Can you work these out from the model? Positions are in its coordinate system, mm. Coordinates: 2 decimals unless noted, no trailing zeros. Order: outer loops, then holes, each group sorted by start corner. A loop starts at its lowest first (then second) coordinate and runs counter-clockwise, first axis right, second up. Notation, with made-up numbers: M 1,-14.75 L 57,-14.75 A31 ccw 57,23.25 Z; hole C 82.5,68.5 d1. An arc over 180 degrees is marked long. Answer as CSV lines item,"result". Start each with the question number.
1. Will this pin go through, and if not, where does the flat tip stop? pin 1 (8 mm diameter, centred on x = -0.5, y = 7.5, fed in from -Z).
2. If we section it at A-A (x = 0): List the corners of the cut face in (y, z) for me, plus the area to 3 significant figures.
3. If we mould it in two halves opening along Y, with no side actions, what happens to faces 1 (the face through (0, -20.5, 3)), 2 (the face through (-10.316, 7.91, 3.328)), 3 (the face through (-14.753, 20.383, 3.328))? For each: released by +Y, released by -Y, zero draft, split by the parting line, or undercut.
4. I need wall thicknesses on line 1 along Y through (x, z) = (0.5, 0.5); line 2 along Y through (x, z) = (16.5, 3); line 3 along Y through (x, z) = (-15.5, 5). Which ranges of each line are inside material? Lowest first, please. Write a range as from..to.
5. If we section it at C-C (z = 5.75): List the corners of the cut face in (x, y) for me.
Autodesk Inventor part; units mm, degrees
ref_plane "Work Plane3" through (0, 0, 0) normal (0, 0, 1) x (1, 0, 0)
ref_plane "YZ Plane" through (0, 0, 0) normal (1, 0, 0) x (0, 1, 0)
ref_plane "XZ Plane" through (0, 0, 0) normal (0, 1, 0) x (-1, 0, 0)
ref_plane "Work Plane3" through (0, 0, 0) normal (0, 0, 1) x (1, 0, 0)
sketch "Sketch1" plane through (0, 0, 0) normal (0, 0, 1) x (1, 0, 0)
  circle A0 centre (15.5, -15.5) radius 1.25
  circle A1 centre (-15.5, -15.5) radius 1.25
  circle A2 centre (15.5, 15.5) radius 1.25
  circle A3 centre (-15.5, 15.5) radius 1.25
  circle A4 centre (0, 0) radius 11
  line L0 (-14.1716, 20.5) -> (14.1716, 20.5)
  arc A5 (-14.1716, 20.5) -> (-15.2322, 20.0607) centre (-14.1716, 19) ccw
  line L1 (-20.0607, 15.2322) -> (-15.2322, 20.0607)
  arc A6 (-20.0607, 15.2322) -> (-20.5, 14.1716) centre (-19, 14.1716) ccw
  line L2 (-20.5, -14.1716) -> (-20.5, 14.1716)
  arc A7 (-20.5, -14.1716) -> (-20.0607, -15.2322) centre (-19, -14.1716) ccw
  line L3 (-15.2322, -20.0607) -> (-20.0607, -15.2322)
  arc A8 (-15.2322, -20.0607) -> (-14.1716, -20.5) centre (-14.1716, -19) ccw
  line L4 (14.1716, -20.5) -> (-14.1716, -20.5)
  arc A9 (14.1716, -20.5) -> (15.2322, -20.0607) centre (14.1716, -19) ccw
  line L5 (20.0607, -15.2322) -> (15.2322, -20.0607)
  arc A10 (20.0607, -15.2322) -> (20.5, -14.1716) centre (19, -14.1716) ccw
  line L6 (20.5, 14.1716) -> (20.5, -14.1716)
  arc A11 (20.5, 14.1716) -> (20.0607, 15.2322) centre (19, 14.1716) ccw
  line L7 (15.2322, 20.0607) -> (20.0607, 15.2322)
  arc A12 (15.2322, 20.0607) -> (14.1716, 20.5) centre (14.1716, 19) ccw
  circle A13 centre (0, 0) radius 13
  circle A14 centre (-15.5, -15.5) radius 1.55
  circle A15 centre (-15.5, 15.5) radius 1.55
  circle A16 centre (15.5, 15.5) radius 1.55
  circle A17 centre (15.5, -15.5) radius 1.55
  point P0 (0, 0)
  dimension "d0" = 2
  dimension "d7" = 3.1
extrude "Extrusion1" add sketch "Sketch1" along normal blind 6.75 contours L0 A12 L7 A11 L6 A10 L5 A9 L4 A8 L3 A7 L2 A6 L1 A5
properties part number "upvulling steppers axis5_6" material "ABS Plastic"
Solved:
1,pin 1,"through"
2,outline,"M -20.5,0 L -13,0 L -13,6.75 L -20.5,6.75 Z; M 13,0 L 20.5,0 L 20.5,6.75 L 13,6.75 Z"
2,area,"101 mm²"
3,face 1,"released by -Y"
3,face 2,"undercut"
3,face 3,"released by +Y"
4,line 1,"-20.5..-12.99, 12.99..20.5"
4,line 2,"-18.79..-16.68, -14.32..14.32, 16.68..18.79"
4,line 3,"-19.79..-17.05, -13.95..13.95, 17.05..19.79"
5,outline,"M -20.5,-14.17 A1.5 ccw -20.06,-15.23 L -15.23,-20.06 A1.5 ccw -14.17,-20.5 L 14.17,-20.5 A1.5 ccw 15.23,-20.06 L 20.06,-15.23 A1.5 ccw 20.5,-14.17 L 20.5,14.17 A1.5 ccw 20.06,15.23 L 15.23,20.06 A1.5 ccw 14.17,20.5 L -14.17,20.5 A1.5 ccw -15.23,20.06 L -20.06,15.23 A1.5 ccw -20.5,14.17 Z; hole C -15.5,-15.5 d3.1; hole C -15.5,15.5 d3.1; hole C 0,0 d26; hole C 15.5,-15.5 d3.1; hole C 15.5,15.5 d3.1"
